from build123d import *

# Parameters (mm, degrees)
F1_DEPTH = 6
F2_R     = 3
F3_DEPTH = 6.001


with BuildPart() as f1:
    # F0 (on Front) → F1 (new body)
    with BuildSketch(Plane.XZ):
        with BuildLine():
            ThreePointArc((2.48542, 12.466661), (2.414328, 13.351159), (2.038464, 14.154973))
            ThreePointArc((2.038464, 14.154973), (1.404844, 14.231831), (0.768425, 14.28034))
            ThreePointArc((0.768425, 14.28034), (0.242655, 13.565528), (0, 12.712))
            ThreePointArc((0, 12.712), (-0.13352, 11.62638), (-0.718152, 10.701931))
            ThreePointArc((-0.718152, 10.701931), (1.053657, 10.674122), (2.796709, 10.354974))
            ThreePointArc((2.796709, 10.354974), (2.404106, 11.375887), (2.48542, 12.466661))
        make_face()
        with BuildLine():
            ThreePointArc((3.431965, 10.16212), (3.11583, 10.263463), (2.796709, 10.354974))
            ThreePointArc((2.796709, 10.354974), (1.053657, 10.674122), (-0.718152, 10.701931))
            ThreePointArc((-0.718152, 10.701931), (-1.049006, 10.67458), (-1.378855, 10.637003))
            ThreePointArc((-1.378855, 10.637003), (-3.111357, 10.26482), (-4.758938, 9.61247))
            ThreePointArc((-4.758938, 9.61247), (-5.05414, 9.460589), (-5.344501, 9.299644))
            ThreePointArc((-5.344501, 9.299644), (-6.802696, 8.292792), (-8.075219, 7.059598))
            ThreePointArc((-8.075219, 7.059598), (-8.289827, 6.806309), (-8.496495, 6.546499))
            ThreePointArc((-8.496495, 6.546499), (-9.458386, 5.058262), (-10.16212, 3.431965))
            ThreePointArc((-10.16212, 3.431965), (-10.263463, 3.11583), (-10.354974, 2.796709))
            ThreePointArc((-10.354974, 2.796709), (-10.674122, 1.053657), (-10.701931, -0.718152))
            ThreePointArc((-10.701931, -0.718152), (-10.67458, -1.049006), (-10.637003, -1.378855))
            ThreePointArc((-10.637003, -1.378855), (-10.26482, -3.111357), (-9.61247, -4.758938))
            ThreePointArc((-9.61247, -4.758938), (-9.460589, -5.05414), (-9.299644, -5.344501))
            ThreePointArc((-9.299644, -5.344501), (-8.292792, -6.802696), (-7.059598, -8.075219))
            ThreePointArc((-7.059598, -8.075219), (-6.806309, -8.289827), (-6.546499, -8.496495))
            ThreePointArc((-6.546499, -8.496495), (-5.058262, -9.458386), (-3.431965, -10.16212))
            ThreePointArc((-3.431965, -10.16212), (-3.11583, -10.263463), (-2.796709, -10.354974))
            ThreePointArc((-2.796709, -10.354974), (-1.053657, -10.674122), (0.718152, -10.701931))
            ThreePointArc((0.718152, -10.701931), (1.049006, -10.67458), (1.378855, -10.637003))
            ThreePointArc((1.378855, -10.637003), (3.111357, -10.26482), (4.758938, -9.61247))
            ThreePointArc((4.758938, -9.61247), (5.05414, -9.460589), (5.344501, -9.299644))
            ThreePointArc((5.344501, -9.299644), (6.802696, -8.292792), (8.075219, -7.059598))
            ThreePointArc((8.075219, -7.059598), (8.289827, -6.806309), (8.496495, -6.546499))
            ThreePointArc((8.496495, -6.546499), (9.458386, -5.058262), (10.16212, -3.431965))
            ThreePointArc((10.16212, -3.431965), (10.263463, -3.11583), (10.354974, -2.796709))
            ThreePointArc((10.354974, -2.796709), (10.632839, -1.410606), (10.726, 0))
            ThreePointArc((10.726, 0), (10.719981, 0.359278), (10.701931, 0.718152))
            ThreePointArc((10.701931, 0.718152), (10.67458, 1.049006), (10.637003, 1.378855))
            ThreePointArc((10.637003, 1.378855), (10.26482, 3.111357), (9.61247, 4.758938))
            ThreePointArc((9.61247, 4.758938), (9.460589, 5.05414), (9.299644, 5.344501))
            ThreePointArc((9.299644, 5.344501), (8.292792, 6.802696), (7.059598, 8.075219))
            ThreePointArc((7.059598, 8.075219), (6.806309, 8.289827), (6.546499, 8.496495))
            ThreePointArc((6.546499, 8.496495), (5.058262, 9.458386), (3.431965, 10.16212))
        make_face()
        with BuildLine():
            ThreePointArc((4.864672, 11.744357), (4.325866, 10.79247), (3.431965, 10.16212))
            ThreePointArc((3.431965, 10.16212), (5.058262, 9.458386), (6.546499, 8.496495))
            ThreePointArc((6.546499, 8.496495), (6.574468, 9.589938), (7.067014, 10.566563))
            ThreePointArc((7.067014, 10.566563), (7.339816, 11.410939), (7.300169, 12.297404))
            ThreePointArc((7.300169, 12.297404), (6.744192, 12.610887), (6.174782, 12.899251))
            ThreePointArc((6.174782, 12.899251), (5.415487, 12.440054), (4.864672, 11.744357))
        make_face()
        with BuildLine():
            ThreePointArc((-4.758938, 9.61247), (-3.111357, 10.26482), (-1.378855, 10.637003))
            ThreePointArc((-1.378855, 10.637003), (-2.132259, 11.429961), (-2.474555, 12.468822))
            ThreePointArc((-2.474555, 12.468822), (-2.878719, 13.258786), (-3.533579, 13.857576))
            ThreePointArc((-3.533579, 13.857576), (-4.14838, 13.686108), (-4.754917, 13.487378))
            ThreePointArc((-4.754917, 13.487378), (-4.967119, 12.625774), (-4.864672, 11.744357))
            ThreePointArc((-4.864672, 11.744357), (-4.57258, 10.690278), (-4.758938, 9.61247))
        make_face()
        with BuildLine():
            ThreePointArc((8.988741, 8.988741), (8.126679, 8.315505), (7.059598, 8.075219))
            ThreePointArc((7.059598, 8.075219), (8.292792, 6.802696), (9.299644, 5.344501))
            ThreePointArc((9.299644, 5.344501), (9.743926, 6.344007), (10.572718, 7.057803))
            ThreePointArc((10.572718, 7.057803), (11.147883, 7.733507), (11.450489, 8.567666))
            ThreePointArc((11.450489, 8.567666), (11.056799, 9.07005), (10.641084, 9.554367))
            ThreePointArc((10.641084, 9.554367), (9.76386, 9.420694), (8.988741, 8.988741))
        make_face()
        with BuildLine():
            ThreePointArc((-8.075219, 7.059598), (-6.802696, 8.292792), (-5.344501, 9.299644))
            ThreePointArc((-5.344501, 9.299644), (-6.344007, 9.743926), (-7.057803, 10.572718))
            ThreePointArc((-7.057803, 10.572718), (-7.733507, 11.147883), (-8.567666, 11.450489))
            ThreePointArc((-8.567666, 11.450489), (-9.07005, 11.056799), (-9.554367, 10.641084))
            ThreePointArc((-9.554367, 10.641084), (-9.420694, 9.76386), (-8.988741, 8.988741))
            ThreePointArc((-8.988741, 8.988741), (-8.315505, 8.126679), (-8.075219, 7.059598))
        make_face()
        with BuildLine():
            ThreePointArc((11.744357, 4.864672), (10.690278, 4.57258), (9.61247, 4.758938))
            ThreePointArc((9.61247, 4.758938), (10.26482, 3.111357), (10.637003, 1.378855))
            ThreePointArc((10.637003, 1.378855), (11.429961, 2.132259), (12.468822, 2.474555))
            ThreePointArc((12.468822, 2.474555), (13.258786, 2.878719), (13.857576, 3.533579))
            ThreePointArc((13.857576, 3.533579), (13.686108, 4.14838), (13.487378, 4.754917))
            ThreePointArc((13.487378, 4.754917), (12.625774, 4.967119), (11.744357, 4.864672))
        make_face()
        with BuildLine():
            ThreePointArc((-10.16212, 3.431965), (-9.458386, 5.058262), (-8.496495, 6.546499))
            ThreePointArc((-8.496495, 6.546499), (-9.589938, 6.574468), (-10.566563, 7.067014))
            ThreePointArc((-10.566563, 7.067014), (-11.410939, 7.339816), (-12.297404, 7.300169))
            ThreePointArc((-12.297404, 7.300169), (-12.610887, 6.744192), (-12.899251, 6.174782))
            ThreePointArc((-12.899251, 6.174782), (-12.440054, 5.415487), (-11.744357, 4.864672))
            ThreePointArc((-11.744357, 4.864672), (-10.79247, 4.325866), (-10.16212, 3.431965))
        make_face()
        with BuildLine():
            ThreePointArc((12.712, 0), (11.62638, 0.13352), (10.701931, 0.718152))
            ThreePointArc((10.701931, 0.718152), (10.719981, 0.359278), (10.726, 0))
            ThreePointArc((10.726, 0), (10.632839, -1.410606), (10.354974, -2.796709))
            ThreePointArc((10.354974, -2.796709), (11.375887, -2.404106), (12.466661, -2.48542))
            ThreePointArc((12.466661, -2.48542), (13.351159, -2.414328), (14.154973, -2.038464))
            ThreePointArc((14.154973, -2.038464), (14.231831, -1.404844), (14.28034, -0.768425))
            ThreePointArc((14.28034, -0.768425), (13.565528, -0.242655), (12.712, 0))
        make_face()
        with BuildLine():
            ThreePointArc((-10.701931, -0.718152), (-10.674122, 1.053657), (-10.354974, 2.796709))
            ThreePointArc((-10.354974, 2.796709), (-11.375887, 2.404106), (-12.466661, 2.48542))
            ThreePointArc((-12.466661, 2.48542), (-13.351159, 2.414328), (-14.154973, 2.038464))
            ThreePointArc((-14.154973, 2.038464), (-14.231831, 1.404844), (-14.28034, 0.768425))
            ThreePointArc((-14.28034, 0.768425), (-13.565528, 0.242655), (-12.712, 0))
            ThreePointArc((-12.712, 0), (-11.62638, -0.13352), (-10.701931, -0.718152))
        make_face()
        with BuildLine():
            ThreePointArc((-9.61247, -4.758938), (-10.26482, -3.111357), (-10.637003, -1.378855))
            ThreePointArc((-10.637003, -1.378855), (-11.429961, -2.132259), (-12.468822, -2.474555))
            ThreePointArc((-12.468822, -2.474555), (-13.258786, -2.878719), (-13.857576, -3.533579))
            ThreePointArc((-13.857576, -3.533579), (-13.686108, -4.14838), (-13.487378, -4.754917))
            ThreePointArc((-13.487378, -4.754917), (-12.625774, -4.967119), (-11.744357, -4.864672))
            ThreePointArc((-11.744357, -4.864672), (-10.690278, -4.57258), (-9.61247, -4.758938))
        make_face()
        with BuildLine():
            ThreePointArc((11.744357, -4.864672), (10.79247, -4.325866), (10.16212, -3.431965))
            ThreePointArc((10.16212, -3.431965), (9.458386, -5.058262), (8.496495, -6.546499))
            ThreePointArc((8.496495, -6.546499), (9.589938, -6.574468), (10.566563, -7.067014))
            ThreePointArc((10.566563, -7.067014), (11.410939, -7.339816), (12.297404, -7.300169))
            ThreePointArc((12.297404, -7.300169), (12.610887, -6.744192), (12.899251, -6.174782))
            ThreePointArc((12.899251, -6.174782), (12.440054, -5.415487), (11.744357, -4.864672))
        make_face()
        with BuildLine():
            ThreePointArc((-7.059598, -8.075219), (-8.292792, -6.802696), (-9.299644, -5.344501))
            ThreePointArc((-9.299644, -5.344501), (-9.743926, -6.344007), (-10.572718, -7.057803))
            ThreePointArc((-10.572718, -7.057803), (-11.147883, -7.733507), (-11.450489, -8.567666))
            ThreePointArc((-11.450489, -8.567666), (-11.056799, -9.07005), (-10.641084, -9.554367))
            ThreePointArc((-10.641084, -9.554367), (-9.76386, -9.420694), (-8.988741, -8.988741))
            ThreePointArc((-8.988741, -8.988741), (-8.126679, -8.315505), (-7.059598, -8.075219))
        make_face()
        with BuildLine():
            ThreePointArc((8.988741, -8.988741), (8.315505, -8.126679), (8.075219, -7.059598))
            ThreePointArc((8.075219, -7.059598), (6.802696, -8.292792), (5.344501, -9.299644))
            ThreePointArc((5.344501, -9.299644), (6.344007, -9.743926), (7.057803, -10.572718))
            ThreePointArc((7.057803, -10.572718), (7.733507, -11.147883), (8.567666, -11.450489))
            ThreePointArc((8.567666, -11.450489), (9.07005, -11.056799), (9.554367, -10.641084))
            ThreePointArc((9.554367, -10.641084), (9.420694, -9.76386), (8.988741, -8.988741))
        make_face()
        with BuildLine():
            ThreePointArc((-3.431965, -10.16212), (-5.058262, -9.458386), (-6.546499, -8.496495))
            ThreePointArc((-6.546499, -8.496495), (-6.574468, -9.589938), (-7.067014, -10.566563))
            ThreePointArc((-7.067014, -10.566563), (-7.339816, -11.410939), (-7.300169, -12.297404))
            ThreePointArc((-7.300169, -12.297404), (-6.744192, -12.610887), (-6.174782, -12.899251))
            ThreePointArc((-6.174782, -12.899251), (-5.415487, -12.440054), (-4.864672, -11.744357))
            ThreePointArc((-4.864672, -11.744357), (-4.325866, -10.79247), (-3.431965, -10.16212))
        make_face()
        with BuildLine():
            ThreePointArc((4.864672, -11.744357), (4.57258, -10.690278), (4.758938, -9.61247))
            ThreePointArc((4.758938, -9.61247), (3.111357, -10.26482), (1.378855, -10.637003))
            ThreePointArc((1.378855, -10.637003), (2.132259, -11.429961), (2.474555, -12.468822))
            ThreePointArc((2.474555, -12.468822), (2.878719, -13.258786), (3.533579, -13.857576))
            ThreePointArc((3.533579, -13.857576), (4.14838, -13.686108), (4.754917, -13.487378))
            ThreePointArc((4.754917, -13.487378), (4.967119, -12.625774), (4.864672, -11.744357))
        make_face()
        with BuildLine():
            ThreePointArc((0.718152, -10.701931), (-1.053657, -10.674122), (-2.796709, -10.354974))
            ThreePointArc((-2.796709, -10.354974), (-2.404106, -11.375887), (-2.48542, -12.466661))
            ThreePointArc((-2.48542, -12.466661), (-2.414328, -13.351159), (-2.038464, -14.154973))
            ThreePointArc((-2.038464, -14.154973), (-1.404844, -14.231831), (-0.768425, -14.28034))
            ThreePointArc((-0.768425, -14.28034), (-0.242655, -13.565528), (0, -12.712))
            ThreePointArc((0, -12.712), (0.13352, -11.62638), (0.718152, -10.701931))
        make_face()
    extrude(amount=F1_DEPTH)

    # F2 (on face) → F3 (cut, through all)
    with BuildSketch(Plane.XZ.offset(6)):
        Circle(F2_R)
    extrude(amount=-F3_DEPTH, mode=Mode.SUBTRACT)


solid = f1.part
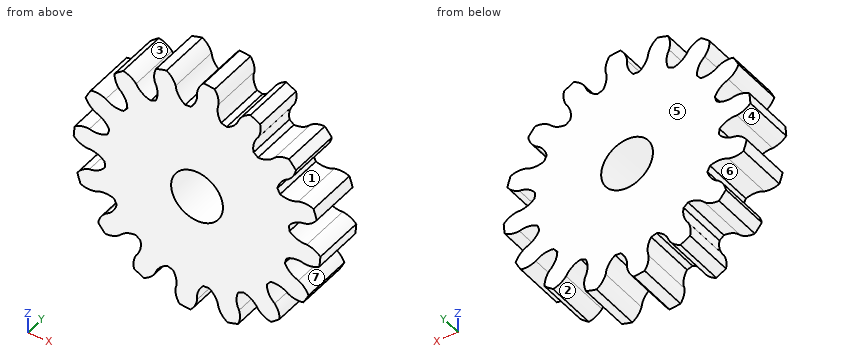
Geometry: final body of the model. Coordinates: model frame, mm. Face numbers are marked on the shaded views. A direction names the side the tool comes from. Give positions to 0.01 mm unless a question says otherwise; leave off trailing zeros. Write each loop counter-clockwise with the first axis right and the second up, starting at its lowest first coordinate (ties: lowest second). Pieces come first, ordered by that corner, then holes. Notation, with made-up numbers: M 78,-13.75 L 118,-13.75 A21 ccw 118,-9.75 Z; hole C 9,16 d4. An arc over 180 degrees is marked long. Answer in a Markdown table with one row per item. Add a question column.
(1) First-contact query: pin 1 (2 mm diameter, centred on x = -10.5, y = -2.5, fed in from -Z); pin 2 (5 mm diameter, centred on x = 0, z = 0, fed in from +Y) (3 decimals); pin 3 (3 mm diameter, centred on y = -3.5, z = -6.5, fed in from +X); pin 4 (2 mm diameter, centred on x = 3, y = -1, fed in from -Z). Flat tips, straight axial feed; report the tip coordinate or a pass-through.
(2) Reachability of the marked faces 1, 2, 3 and 4 from +Z, -Z, +X, -X, +Y, -Y: full face, straight path, thin tool, end or side. Return the list, or none.
(3) Mould query, pull axis X, two halves, no side actions, for the marked faces 5, 6 and 7. Classes: +X half, -X half, draft (parallel to the pull), parting line (faces both ways), or undercut.
(4) Ray query, line 1 (X direction, y = -5.2, z = -11); line 2 (X direction, y = -4.3, z = 12.75); line 3 (Z direction, x = 13, y = -1.3). Return the intervals inside material, ascending.
(5) Section A-A on z = -4. Return loops of the section in (x, y), and give its area (3 significant figures).
Result set:
| question | item | result |
|---|---|---|
| 1 | pin 1 | stops at z = -9.56 |
| 1 | pin 2 | passes through |
| 1 | pin 3 | stops at x = 12.9 |
| 1 | pin 4 | stops at z = -13.86 |
| 2 | face 1 | +Y, -Y |
| 2 | face 2 | -Z, +Y, -Y |
| 2 | face 3 | +Z, +Y, -Y |
| 2 | face 4 | -X, +Y, -Y |
| 3 | face 5 | draft |
| 3 | face 6 | undercut |
| 3 | face 7 | +X half |
| 4 | line 1 | x = -7.25 to -4.49, -2.49 to 0.46, 1.81 to 4.61, 7.51 to 9.14 |
| 4 | line 2 | x = -4.96 to -2.58, 0 to 2.5, 5.85 to 6.48 |
| 4 | line 3 | z = -2.48 to -0.05, 2.71 to 4.91 |
| 5 | outline | M -13.73,-6 L 10.49,-6 L 10.49,0 L -13.73,0 Z |
| 5 | area | 145 mm^2 |
